For this review, take the finished solid that the model builds, in its own axes (mm). Face numbers are marked on the shaded views. Round coordinates to 2 decimals unless told otherwise and drop trailing zeros. Order: outer loops, then holes, each group sorted by start corner. A loop starts at its lowest first (then second) coordinate and runs counter-clockwise, first axis right, second up. Notation, with made-up numbers: M 7.25,11.5 L 29.25,11.5 A32 cw 29.25,43.5 Z; hole C -24.5,-8 d10. An arc over 180 degrees is marked long. Put each result on its own line as item: value.
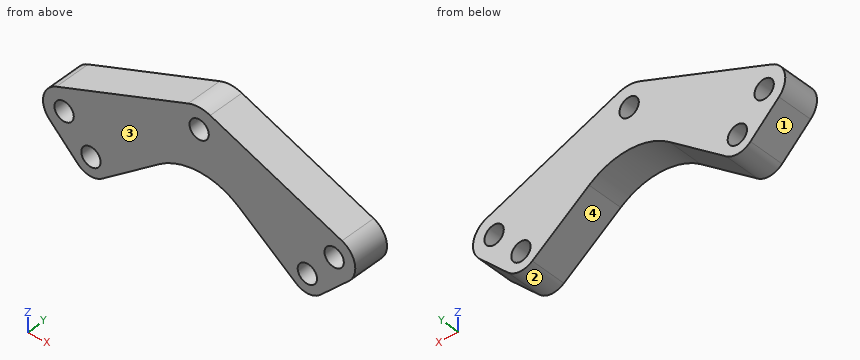
from build123d import *

# Parameters (mm, degrees)
ESBO_O1_R                = 1.6
RESSALTO_EXTRUS_O1_DEPTH = 6


with BuildPart() as part:
    # Esboço1 → Ressalto-extrusão1 (new body)
    with BuildSketch(Plane.XZ.offset(6)):
        with BuildLine():
            Line((23.658239146, -5.419790473), (1.830835365, 3.169198905))
            ThreePointArc((1.830835365, 3.169198905), (0, 3.516453278), (-1.830835365, 3.169198905))
            Line((-1.830835365, 3.169198905), (-23.658239146, -5.419790473))
            ThreePointArc((-23.658239146, -5.419790473), (-25.806836409, -7.98111819), (-24.825744035, -11.177104364))
            Line((-24.825744035, -11.177104364), (-20.101514858, -15.804403192))
            ThreePointArc((-20.101514858, -15.804403192), (-18.128320556, -16.683568025), (-16.059952818, -16.060445681))
            Line((-16.059952818, -16.060445681), (-6.643887712, -8.924606384))
            ThreePointArc((-6.643887712, -8.924606384), (0, -6.691518958), (6.643887712, -8.924606384))
            Line((6.643887712, -8.924606384), (16.059952818, -16.060445681))
            ThreePointArc((16.059952818, -16.060445681), (18.128320556, -16.683568025), (20.101514858, -15.804403192))
            Line((20.101514858, -15.804403192), (24.825744035, -11.177104364))
            ThreePointArc((24.825744035, -11.177104364), (25.806836409, -7.98111819), (23.658239146, -5.419790473))
        make_face()
        with Locations(Location((-17.932321173, -13.589770319, 0), (0, 0, 90))):
            Circle(ESBO_O1_R, mode=Mode.SUBTRACT)
        with Locations(Location((0, 0, 0), (0, 0, 90))):
            Circle(ESBO_O1_R, mode=Mode.SUBTRACT)
        with Locations(Location((17.932321173, -13.589770319, 0), (0, 0, 90))):
            Circle(ESBO_O1_R, mode=Mode.SUBTRACT)
        with Locations(Location((-22.376654391, -8.676712411, 0), (0, 0, 90))):
            Circle(ESBO_O1_R, mode=Mode.SUBTRACT)
        with Locations(Location((22.376654391, -8.676712411, 0), (0, 0, 90))):
            Circle(ESBO_O1_R, mode=Mode.SUBTRACT)
    extrude(amount=-RESSALTO_EXTRUS_O1_DEPTH)


solid = part.part
(1) Draft analysis for pull direction X (two halves, no side actions). For the marked faces 1, 2, 3 and 4, state which applies: released by +X, released by -X, zero draft, split by the parting line, or undercut.
A:
face 1: released by -X
face 2: undercut
face 3: zero draft
face 4: undercut
(2) Add section D-D on x = 5.5. Give the boundary of the cut face in (y, z).
A:
outline: M -6,-8.17 L 0,-8.17 L 0,1.73 L -6,1.73 Z
(3) Add section A-A on x = 0. Give the boundary of the cut face in (y, z), then the cut area to 3 significant figures.
A:
outline: M -6,-6.69 L 0,-6.69 L 0,-1.6 L -6,-1.6 Z; M -6,1.6 L 0,1.6 L 0,3.52 L -6,3.52 Z
area: 42.0 mm2
(4) Insertion check: pin 1 Ø1.9 at (x, z) = (22.38, -8.68) entering from -Y; pin 2 Ø1 at (x, y) = (-8.5, -3) entering from +Z. Each pin has a flat end and moves straight along its axis. Give the tip position at first contact, or say it passes through.
A:
pin 1: passes through
pin 2: stops at z = 0.74
(5) Add section C-C on y = -2.05. Give the boundary of the cut face in (x, z), then the cut area to 3 significant figures.
A:
outline: M -24.83,-11.18 L -20.1,-15.8 A3.1 ccw -16.06,-16.06 L -6.64,-8.92 A11 cw 6.64,-8.92 L 16.06,-16.06 A3.1 ccw 20.1,-15.8 L 24.83,-11.18 A3.5 ccw 23.66,-5.42 L 1.83,3.17 A5 ccw -1.83,3.17 L -23.66,-5.42 A3.5 ccw Z; hole C -22.38,-8.68 d3.2; hole C -17.93,-13.59 d3.2; hole C 0,0 d3.2; hole C 17.93,-13.59 d3.2; hole C 22.38,-8.68 d3.2
area: 511 mm2
(6) To check wall thickness, follow L1, parallel to X at y = -1.45, z = -9.5; L2, parallel to X at y = -5.05, z = -13.5; L3, parallel to Z at x = -19, y = -3.5. State the ranges of each line that lie inside material, in increasing order.
A:
L1: x = -25.78 to -23.75, -21 to -7.4, 7.4 to 21, 23.75 to 25.78
L2: x = -22.45 to -19.53, -16.33 to -12.68, 12.68 to 16.33, 19.53 to 22.45
L3: z = -16.5 to -14.78, -12.4 to -3.59
(7) Add section B-B on z = 0. Give the boundary of the cut face in (x, y), then the cut area to 3 significant figures.
A:
outline: M -9.88,-6 L -1.6,-6 L -1.6,0 L -9.88,0 Z; M 1.6,-6 L 9.88,-6 L 9.88,0 L 1.6,0 Z
area: 99.4 mm2
